Geometry check sheet. Reference: the model listing, model coordinates, mm. A direction names the side the tool comes from. Round coordinates to 2 decimals unless told otherwise and drop trailing zeros. Loops run counter-clockwise (first coordinate to the right, second up) from the corner with the lowest first, then second, coordinate; pieces in that order, holes last.
```python
from build123d import *

# Parameters (mm, degrees)
SKETCH1_R                      = 40
BOSS_EXTRUDE1_DEPTH            = 50
SKETCH2_R                      = 10.425
CUT_EXTRUDE1_DEPTH             = 30
SKETCH3_R                      = 20
SKETCH3_R_2                    = 10
CUT_EXTRUDE2_DEPTH             = 5
SKETCH5_R                      = 2.5
CUT_EXTRUDE4_DEPTH             = 76.498344353
SKETCH4_R                      = 0.5
CUT_EXTRUDE6_DEPTH             = 76.498344353
CUT_EXTRUDE7_REACH             = 77.498
SKETCH7_R                      = 1.25
CUT_EXTRUDE7_DIRECTION_2_REACH = 77.498


with BuildPart() as part:
    # Sketch1 → Boss-Extrude1 (new body)
    with BuildSketch(Plane(origin=(0, 0, 0), x_dir=(0, 0, -1), z_dir=(1, 0, 0))):
        Circle(SKETCH1_R)
    extrude(amount=BOSS_EXTRUDE1_DEPTH)

    # Sketch2 → Cut-Extrude1 (cut)
    with BuildSketch(Plane(origin=(50, 0, 0), x_dir=(0, 0, -1), z_dir=(1, 0, 0))):
        Circle(SKETCH2_R)
    extrude(amount=-CUT_EXTRUDE1_DEPTH, mode=Mode.SUBTRACT)

    # Sketch3 → Cut-Extrude2 (cut)
    with BuildSketch(Plane.ZY):
        Circle(SKETCH3_R)
        Circle(SKETCH3_R_2, mode=Mode.SUBTRACT)
    extrude(amount=-CUT_EXTRUDE2_DEPTH, mode=Mode.SUBTRACT)

    # Sketch5 → Cut-Extrude4 (cut, through all)
    with BuildSketch(Plane.ZY):
        with Locations((0, 30)):
            Circle(SKETCH5_R)
        with Locations((30, 0)):
            Circle(SKETCH5_R)
        with Locations((0, -30)):
            Circle(SKETCH5_R)
        with Locations((-30, 0)):
            Circle(SKETCH5_R)
    extrude(amount=-CUT_EXTRUDE4_DEPTH, mode=Mode.SUBTRACT)

    # Sketch8 → Revolve4 (revolve)
    with BuildSketch(Plane.XY, mode=Mode.PRIVATE) as revolve4_sk:
        Polygon((27.456013161, 12.408889724), (20.184130796, 0.306445106), (19.15133868, 0.306445106), (19.15133868, 12.408889724), align=None)
    revolve(revolve4_sk.sketch.rotate(Axis((-60.024183688, 0, 0), (1, 0, 0)), 270), axis=Axis((-60.024183688, 0, 0), (1, 0, 0)))

    # Sketch4 → Cut-Extrude6 (cut, through all)
    with BuildSketch(Plane.ZY):
        Circle(SKETCH4_R)
    extrude(amount=-CUT_EXTRUDE6_DEPTH, mode=Mode.SUBTRACT)

    # Sketch7 → Cut-Extrude7 (cut, up to next)
    with BuildSketch(Plane(origin=(0, 0, 0), x_dir=(0, 0, 1), z_dir=(-0.9063077870366495, 0.4226182617407003, 0)), mode=Mode.PRIVATE) as cut_extrude7_sk1:
        with Locations(Location((0, 12.678547852, 0), (0, 0, 258.66668262))):
            Circle(SKETCH7_R)
    cut_extrude7_tool1 = extrude(cut_extrude7_sk1.sketch, amount=-CUT_EXTRUDE7_REACH, mode=Mode.PRIVATE) & part.part
    cut_extrude7 = cut_extrude7_tool1.solids().sort_by_distance((5.358186, 11.490667, 0))[0]
    add(cut_extrude7, mode=Mode.SUBTRACT)

    # Sketch7 → Cut-Extrude7 direction 2 (cut, up to next)
    with BuildSketch(Plane(origin=(0, 0, 0), x_dir=(0, 0, 1), z_dir=(-0.9063077870366495, 0.4226182617407003, 0)), mode=Mode.PRIVATE) as cut_extrude7_direction_2_sk1:
        with Locations(Location((0, 12.678547852, 0), (0, 0, 258.66668262))):
            Circle(SKETCH7_R)
    cut_extrude7_direction_2_tool1 = extrude(cut_extrude7_direction_2_sk1.sketch, amount=CUT_EXTRUDE7_DIRECTION_2_REACH, mode=Mode.PRIVATE) & part.part
    cut_extrude7_direction_2 = cut_extrude7_direction_2_tool1.solids().sort_by_distance((5.358186, 11.490667, 0))[0]
    add(cut_extrude7_direction_2, mode=Mode.SUBTRACT)

    # Mirror1: Cut-Extrude7, Cut-Extrude7 direction 2 across plane
    add(cut_extrude7.mirror(Plane.ZX), mode=Mode.SUBTRACT)
    add(cut_extrude7_direction_2.mirror(Plane.ZX), mode=Mode.SUBTRACT)


solid = part.part
```
1) Scan lines: line 1 along Y through (x, z) = (32.5, 0) (3 decimals); line 2 along Z through (x, y) = (40.5, -5); line 3 along Y through (x, z) = (9.5, 31). Record each from-to range of solid material in increasing order.
Report:
line 1: y = -40 to -32.5, -27.5 to -10.425, 10.425 to 27.5, 32.5 to 40
line 2: z = -39.69 to -9.15, 9.15 to 39.69
line 3: y = -25.28 to -2.29, 2.29 to 25.28
2) Sectioned sample at C-C, the plane z = -30. Record the cut outline in (x, y).
Report:
outline: (0, -26.46) - (50, -26.46) - (50, -2.5) - (0, -2.5) - close; (0, 2.5) - (50, 2.5) - (50, 26.46) - (0, 26.46) - close
3) Sectioned sample at B-B, the plane x = 35. Record the cut outline in (y, z) (3 decimals), then the cut area to 3 significant figures.
Report:
outline: circle Ø80 at (0, 0); hole circle Ø5 at (-30, 0); hole circle Ø20.85 at (0, 0); hole circle Ø5 at (0, -30); hole circle Ø5 at (0, 30); hole circle Ø5 at (30, 0)
area: 4,610 mm2
4) Gauge pin test, flat ends, axial feed: pin 1 (10 mm diameter, centred on x = 19, y = -21, fed in from +Z); pin 2 (3 mm diameter, centred on y = 1, z = 2.5, fed in from +X); pin 3 (10 mm diameter, centred on x = 29, z = -6.5, fed in from -Y); pin 4 (4 mm diameter, centred on y = 0, z = -30, fed in from -X). Record the tip position at first contact, or that the pin passes through.
Report:
pin 1: stops at z = 36.66
pin 2: stops at x = 22.52
pin 3: stops at y = -39.97
pin 4: passes through
5) Sectioned sample at A-A, the plane y = 29. Record the cut outline in (x, z), then the cut area to 3 significant figures.
Report:
outline: (0, -27.55) - (50, -27.55) - (50, -2.29) - (0, -2.29) - close; (0, 2.29) - (50, 2.29) - (50, 27.55) - (0, 27.55) - close
area: 2,530 mm2
6) Sectioned sample at D-D, the plane y = -34. Record the cut outline in (x, z).
Report:
outline: (0, -21.07) - (50, -21.07) - (50, 21.07) - (0, 21.07) - close
7) Mould release check, pull along Y, two halves, no side actions. Record for faces 4 (the face through (24.6, 0.1, -32.5)), 5 (the face through (24.65, -39.05, 8.67)), 6 (the face through (0, 0, -2)): +Y half, -Y half, draft (parallel to the pull), parting line (faces both ways), or undercut.
Report:
face 4: undercut
face 5: parting line
face 6: draft
8) Access from +Z, -Z, +X, -X, +Y, -Y to the whole of each face (thin tool, end or side, straight path). Record for faces 1 (the face through (38.298, 3.131, -9.944)), 2 (the face through (13.781, -8.902, 0.299)), 3 (the face through (2.46, -9.76, -2.17)).
Report:
face 1: +X
face 2: none
face 3: -X
